Geometry: see drawing. Coordinates: mm, zero at the bounding-box minimum. A direction names the side the tool comes from. Give positions to 0.01 mm unless a question says otherwise; leave off trailing zeros. Loops run counter-clockwise (first coordinate to the right, second up) from the corner with the lowest first, then second, coordinate; pieces in that order, holes last. Notation, with made-up numbers: (25, 80) -> (68, 80) arc R14 ccw to (68, 91) -> close; hole circle Ø5 at (21, 26). An arc over 180 degrees is marked (long way). One line per question, with ' | ' between items.
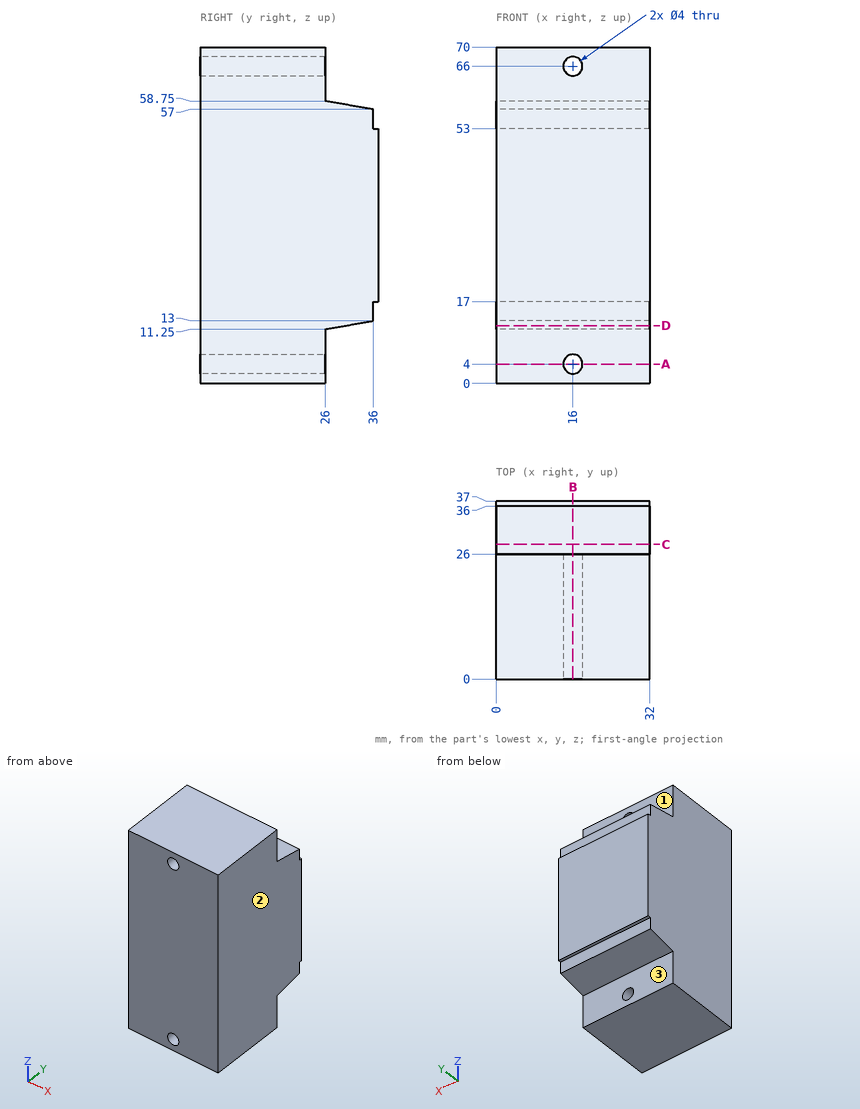
1. Section query B-B (x = 16). Output: boundary loops of the cut face in (y, z).
Determined:
outline: (0, 0) -> (26, 0) -> (26, 2) -> (0, 2) -> close; (0, 6) -> (26, 6) -> (26, 11.25) -> (36, 13) -> (36, 17) -> (37, 17) -> (37, 53) -> (36, 53) -> (36, 57) -> (26, 58.75) -> (26, 64) -> (0, 64) -> close; (0, 68) -> (26, 68) -> (26, 70) -> (0, 70) -> close
2. Reachability of the marked faces 1, 2 and 3 from +Z, -Z, +X, -X, +Y, -Y: full face, straight path, thin tool, end or side. Return the list, or none.
Determined:
face 1: +Z, +X, -X, +Y | face 2: +Z, -Z, +X, +Y, -Y | face 3: -Z, +X, -X, +Y
3. Ray query, line 1 along X through (y, z) = (5.75, 66); line 2 along Z through (x, y) = (17, 17.5); line 3 along Y through (x, z) = (22, 61). Return the intervals inside material, ascending. Write a range as from..to.
Determined:
line 1: x = 0..14, 18..32 | line 2: z = 0..2.27, 5.73..64.27, 67.73..70 | line 3: y = 0..26
4. Section query C-C (y = 28). Output: boundary loops of the cut face in (x, z).
Determined:
outline: (0, 11.6) -> (32, 11.6) -> (32, 58.4) -> (0, 58.4) -> close
5. Section query A-A (z = 4). Output: boundary loops of the cut face in (x, y).
Determined:
outline: (0, 0) -> (14, 0) -> (14, 26) -> (0, 26) -> close; (18, 0) -> (32, 0) -> (32, 26) -> (18, 26) -> close
6. Section query D-D (z = 12). Output: boundary loops of the cut face in (x, y), then the cut area to 3 significant figures.
Determined:
outline: (0, 0) -> (32, 0) -> (32, 30.29) -> (0, 30.29) -> close | area: 969 mm2
7. Pin query (flat end, axial travel): P1, Ø8, axis at x = 22.5, y = 29.5, coming from the -Z side; P2, Ø12, axis at x = 4.5, y = 33, coming from the +Z side (3 decimals); P3, Ø12.5, axis at x = 14.5, z = 66, coming from the +Y side; P4, Ø1.2, axis at x = 15, z = 15.5, coming from the +Y side. Return the tip coordinate at first contact, or that it passes through.
Determined:
P1: stops at z = 0 | P2: stops at z = 58.575 | P3: stops at y = 26 | P4: stops at y = 36
